from build123d import *

# Parameters (mm, degrees)
SKETCH1_W           = 203.2
SKETCH1_H           = 203.2
BOSS_EXTRUDE1_DEPTH = 22.225
CUT_EXTRUDE1_START  = -203.2
CUT_EXTRUDE1_DEPTH  = 203.2
SKETCH3_R           = 88.9
BOSS_EXTRUDE2_DEPTH = 31.75
SKETCH4_R           = 51.25
CUT_EXTRUDE2_DEPTH  = 290.116832062
CIRPATTERN1_COUNT   = 8
CIRPATTERN2_COUNT   = 8


# Read off the part's stored shape, not the designer's step: Cut-Extrude1
with BuildPart() as part:
    # Sketch1 → Boss-Extrude1 (new body)
    with BuildSketch(Plane(origin=(0, 0, 0), x_dir=(1, 0, 0), z_dir=(0, 1, 0))):
        with Locations((101.6, 101.6)):
            Rectangle(SKETCH1_W, SKETCH1_H)
    extrude(amount=BOSS_EXTRUDE1_DEPTH)

    # Cut-Extrude1 outline → Cut-Extrude1 (cut)
    with BuildSketch(Plane.XY.offset(CUT_EXTRUDE1_START)):
        with BuildLine():
            ThreePointArc((0, 12.339521695), (50.560108139, 19.747808997), (101.600002148, 22.225))
            Line((101.600002148, 22.225), (0, 22.225))
            Line((0, 22.225), (0, 12.339521695))
        make_face()
        with BuildLine():
            ThreePointArc((101.600002148, 22.225), (152.639893999, 19.747808789), (203.2, 12.339521695))
            Line((203.2, 12.339521695), (203.2, 22.225))
            Line((203.2, 22.225), (101.600002148, 22.225))
        make_face()
    extrude(amount=CUT_EXTRUDE1_DEPTH, mode=Mode.SUBTRACT)

    # Sketch3 → Boss-Extrude2 (add)
    with BuildSketch(Plane(origin=(0, 0, 0), x_dir=(-1, 0, 0), z_dir=(0, -1, 0))):
        with Locations(Location((-101.6, 101.6, 0), (0, 0, 90))):
            Circle(SKETCH3_R)
    extrude(amount=-BOSS_EXTRUDE2_DEPTH)

    # Sketch4 → Cut-Extrude2 (cut, through all)
    with BuildSketch(Plane(origin=(0, 31.75, 0), x_dir=(1, 0, 0), z_dir=(0, 1, 0))):
        with Locations(Location((101.6, 101.6, 0), (0, 0, 270))):
            Circle(SKETCH4_R)
    extrude(amount=-CUT_EXTRUDE2_DEPTH, mode=Mode.SUBTRACT)

    # Sketch6 → Tapped Hole for 5/16-18 Helicoil1 (revolve, cut)
    with BuildSketch(Plane(origin=(101.6, 31.75, -174.1), x_dir=(0, 0, 1), z_dir=(1, 0, 0))):
        Polygon((0, 0), (0, 22.878868714), (4.2164, 20.3454), (4.2164, 0), align=None)
    tapped_hole_for_5_16_18_helicoil1 = revolve(axis=Axis((101.6, 38.1, -174.1), (0, -1, 0)), mode=Mode.SUBTRACT)

    # CirPattern1: Tapped Hole for 5/16-18 Helicoil1 ×8 about axis
    cirpattern1_axis = Axis((101.6, 0, -101.6), (0, 1, 0))
    for i in range(1, CIRPATTERN1_COUNT):
        add(tapped_hole_for_5_16_18_helicoil1.rotate(cirpattern1_axis, i * 360 / CIRPATTERN1_COUNT), mode=Mode.SUBTRACT)

    # Sketch13 → Tapped Hole for 5/16-18 Helicoil2 (revolve, cut)
    with BuildSketch(Plane(origin=(129.344548846, 0, -34.618733893), x_dir=(0, 0, -1), z_dir=(1, 0, 0))):
        Polygon((0, 0), (0, 22.878868714), (4.2164, 20.3454), (4.2164, 0), align=None)
    tapped_hole_for_5_16_18_helicoil2 = revolve(axis=Axis((129.344548846, -6.35, -34.618733893), (0, 1, 0)), mode=Mode.SUBTRACT)

    # CirPattern2: Tapped Hole for 5/16-18 Helicoil2 ×8 about axis
    cirpattern2_axis = Axis((101.6, 0, -101.6), (0, 1, 0))
    for i in range(1, CIRPATTERN2_COUNT):
        add(tapped_hole_for_5_16_18_helicoil2.rotate(cirpattern2_axis, i * 360 / CIRPATTERN2_COUNT), mode=Mode.SUBTRACT)


solid = part.part
Input: part model. Units: mm. Frame: model coordinates. A direction names the side the tool comes from. Round coordinates to 2 decimals unless told otherwise and drop trailing zeros. Loops run counter-clockwise (first coordinate to the right, second up) from the corner with the lowest first, then second, coordinate; pieces in that order, holes last. Notation, with made-up numbers: (-33.5, 50) -> (25.5, 50) arc R6 cw to (25.5, 54) -> close; hole circle Ø7 at (-3.75, 65.25). An arc over 180 degrees is marked (long way). Answer as a JSON object with one key per item and string values. Group by question number.
1) Section query C-C on x = 43. Output: boundary loops of the cut face in (y, z).
2) Section query A-A on z = -144.5. Output: boundary loops of the cut face in (x, y) (3 decimals).
3) Section query D-D on z = -41.5. Output: boundary loops of the cut face in (x, y) (3 decimals), plus the area to 3 significant figures.
4) Pin query (flat end, axial travel): pin 1 (6.5 mm diameter, centred on x = 101.6, z = -174.1, fed in from +Y); pin 2 (12 mm diameter, centred on y = 22, z = -115, fed in from -X); pin 3 (6.5 mm diameter, centred on x = 73.86, z = -168.58, fed in from -Y). Return the tip coordinate at first contact, or that it passes through.
5) Draft query along Z for faces 4 (the flat face through (148, 0, -78)), 5 (the conical face through (50.303, 9.311, -49.603)), 6 (the flat face through (100, 8, -203.2)). Return one class per face: +Z half, -Z half, draft (parallel to the pull), parting line (faces both ways), or undercut.
6) Section query B-B on y = 28.5. State how many separate pieces and enclosed holes the cut face has, plus the area to 3 significant figures.
7) Reachability of faces 1 (the flat face through (63, 31.75, -140)), 2 (the cylindrical face through (102.87, 21.72, -33.12)), 3 (the cylindrical face through (75.8, 10.03, -38.36)) from +Z, -Z, +X, -X, +Y, -Y: full face, straight path, thin tool, end or side. Return the list, or none.
8) Ray query, L1, parallel to X at y = 3, z = -38; L2, parallel to Z at x = 29, y = 10.5; L3, parallel to Z at x = 117, y = 26.5. Return the intervals inside material, ascending.
Reply:
{
 "1": {"outline": "(0, -203.2) -> (18.96, -203.2) -> (18.96, -168.45) -> (31.75, -168.45) -> (31.75, -34.75) -> (18.96, -34.75) -> (18.96, 0) -> (0, 0) -> close"},
 "2": {"outline": "(0, 0) -> (73.562, 0) -> (73.562, 31.75) -> (23.736, 31.75) -> (23.736, 16.442) arc R527.05 ccw to (0, 12.34) -> close; (129.638, 0) -> (203.2, 0) -> (203.2, 12.34) arc R527.05 ccw to (179.464, 16.442) -> (179.464, 31.75) -> (129.638, 31.75) -> close"},
 "3": {"outline": "(0, 0) -> (203.2, 0) -> (203.2, 12.34) arc R527.05 ccw to (167.107, 18.138) -> (167.107, 31.75) -> (36.093, 31.75) -> (36.093, 18.138) arc R527.05 ccw to (0, 12.34) -> close", "area": "5,280 mm2"},
 "4": {"pin 1": "stops at y = 10.82", "pin 2": "stops at x = 13.01", "pin 3": "stops at y = 20.92"},
 "5": {"face 4": "draft", "face 5": "undercut", "face 6": "-Z half"},
 "6": {"separate pieces": "1", "enclosed holes": "9", "area": "16,100 mm2"},
 "7": {"face 1": "+Z, -Z, +X, -X, +Y", "face 2": "+Y", "face 3": "-Y"},
 "8": {"L1": "x = 0 to 71.34, 76.37 to 126.83, 131.86 to 203.2", "L2": "z = -203.2 to -104.31, -98.89 to 0", "L3": "z = -189.16 to -150.48, -52.72 to -14.04"}
}
